Could you check a few things on this model? Use its own coordinates, in mm. Face numbers are marked on the shaded views. A direction names the side the tool comes from. Give positions to 0.01 mm unless a question says otherwise; leave off trailing zeros. Order: outer loops, then holes, each group sorted by start corner. A loop starts at its lowest first (then second) coordinate and runs counter-clockwise, first axis right, second up.
from build123d import *

# Parameters (mm, degrees)
SZKIC1_W                        = 27
SZKIC1_H                        = 25
ZAOKR_GLENIE1_R                 = 4
SZKIC4_R                        = 3
WYTNIJ_WYCI_GNI_CIE3_DEPTH      = 24.0000001
WYTNIJ_WYCI_GNI_CIE3_DEPTH_BACK = 3
WYTNIJ_WYCI_GNI_CIE2_DEPTH      = 24.0000001
SZKIC5_OUTSIDE_W                = 72.072
SZKIC5_OUTSIDE_H                = 72.072
WYTNIJ_WYCI_GNI_CIE4_DEPTH      = 26.0000001
SZKIC6_R                        = 2.675
WYTNIJ_WYCI_GNI_CIE5_DEPTH      = 26.0000001
SZKIC7_OUTSIDE_W                = 68.298
SZKIC7_OUTSIDE_H                = 29.798
WYTNIJ_WYCI_GNI_CIE6_DEPTH      = 5.5


with BuildPart() as part:
    # Szkic1 → Obrót1 (revolve)
    with BuildSketch(Plane.XY):
        with Locations((13.5, 12.5)):
            Rectangle(SZKIC1_W, SZKIC1_H)
    revolve(axis=Axis((0, 0, 0), (0, 1, 0)))

    # Szkic2 → Wycięcie-obrót1 (revolve, cut)
    with BuildSketch(Plane.XY):
        Polygon((5.55, 25), (5.55, 14.384163274), (27, 2), (27, 25), align=None)
    revolve(axis=Axis((0, 0, 0), (0, 1, 0)), mode=Mode.SUBTRACT)

    # Zaokrąglenie1
    zaokr_glenie1_edges = [part.edges().sort_by_distance(p)[0] for p in [
        (-5.55, 14.384163274, 0),
    ]]
    fillet(zaokr_glenie1_edges, radius=ZAOKR_GLENIE1_R)

    # Szkic4 → Wytnij-wyciągnięcie3 (cut, two sides)
    with BuildSketch(Plane(origin=(0, 2, 0), x_dir=(1, 0, 0), z_dir=(0, 1, 0))) as wytnij_wyci_gni_cie3_sk:
        with Locations((-20, 0)):
            Circle(SZKIC4_R)
        with Locations((20, 0)):
            Circle(SZKIC4_R)
    extrude(amount=WYTNIJ_WYCI_GNI_CIE3_DEPTH, mode=Mode.SUBTRACT)
    extrude(wytnij_wyci_gni_cie3_sk.sketch, amount=-WYTNIJ_WYCI_GNI_CIE3_DEPTH_BACK, mode=Mode.SUBTRACT)

    # Szkic3 → Wytnij-wyciągnięcie2 (cut, through all)
    with BuildSketch(Plane(origin=(0, 2, 0), x_dir=(1, 0, 0), z_dir=(0, 1, 0))):
        with BuildLine():
            Line((-17.5, 5), (-26.532998323, 5))
            ThreePointArc((-26.532998323, 5), (-27, 0), (-26.532998323, -5))
            Line((-26.532998323, -5), (-17.5, -5))
            ThreePointArc((-17.5, -5), (-12.5, 0), (-17.5, 5))
        make_face()
        with BuildLine():
            Line((17.5, 5), (26.532998323, 5))
            ThreePointArc((26.532998323, 5), (27, 0), (26.532998323, -5))
            Line((26.532998323, -5), (17.5, -5))
            ThreePointArc((17.5, -5), (12.5, 0), (17.5, 5))
        make_face()
    extrude(amount=WYTNIJ_WYCI_GNI_CIE2_DEPTH, mode=Mode.SUBTRACT)

    # Szkic5 outside → Wytnij-wyciągnięcie4 (cut, through all)
    with BuildSketch(Plane.XZ):
        Rectangle(SZKIC5_OUTSIDE_W, SZKIC5_OUTSIDE_H)
        with BuildLine():
            Line((-20.2625, 6.995076393), (-0.290625, 7.744548864))
            ThreePointArc((-0.290625, 7.744548864), (0, 7.75), (0.290625, 7.744548864))
            Line((0.290625, 7.744548864), (20.2625, 6.995076393))
            ThreePointArc((20.2625, 6.995076393), (27, 0), (20.2625, -6.995076393))
            Line((20.2625, -6.995076393), (0.290625, -7.744548864))
            ThreePointArc((0.290625, -7.744548864), (0, -7.75), (-0.290625, -7.744548864))
            Line((-0.290625, -7.744548864), (-20.2625, -6.995076393))
            ThreePointArc((-20.2625, -6.995076393), (-27, 0), (-20.2625, 6.995076393))
        make_face(mode=Mode.SUBTRACT)
    extrude(amount=-WYTNIJ_WYCI_GNI_CIE4_DEPTH, mode=Mode.SUBTRACT)

    # Szkic6 → Wytnij-wyciągnięcie5 (cut, through all)
    with BuildSketch(Plane(origin=(0, 25, 0), x_dir=(1, 0, 0), z_dir=(0, 1, 0))):
        Circle(SZKIC6_R)
    extrude(amount=-WYTNIJ_WYCI_GNI_CIE5_DEPTH, mode=Mode.SUBTRACT)

    # Szkic7 outside → Wytnij-wyciągnięcie6 (cut)
    with BuildSketch(Plane(origin=(0, 25, 0), x_dir=(1, 0, 0), z_dir=(0, 1, 0))):
        Rectangle(SZKIC7_OUTSIDE_W, SZKIC7_OUTSIDE_H)
        Polygon((-4.806440991, 2.775), (-4.806440991, -2.775), (0, -5.55), (4.806440991, -2.775), (4.806440991, 2.775), (0, 5.55), align=None, mode=Mode.SUBTRACT)
    extrude(amount=-WYTNIJ_WYCI_GNI_CIE6_DEPTH, mode=Mode.SUBTRACT)

    # Szkic9 → Wycięcie-obrót2 (revolve, cut)
    with BuildSketch(Plane.XY):
        Polygon((4.05, 25), (5.55, 24.133974596), (5.55, 25), align=None)
    revolve(axis=Axis((0, 19.5, 0), (0, 1, 0)), mode=Mode.SUBTRACT)


solid = part.part
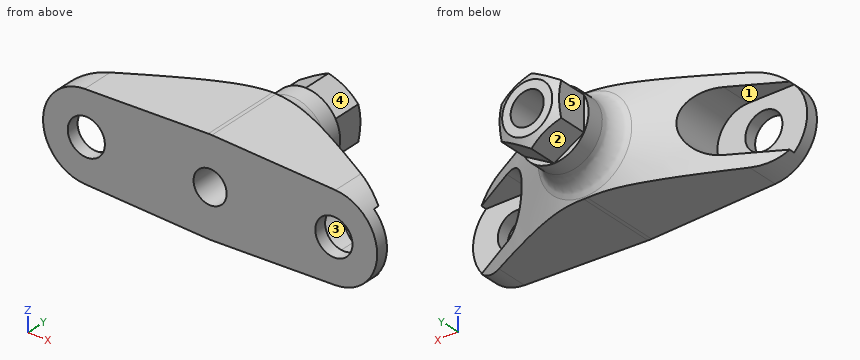
Item 1: For the marked faces 1, 2, 3, 4 and 5, which set-ups out of +Z, -Z, +X, -X, +Y, -Y let a thin tool reach every point of the face, with its end or its side?
Findings:
face 1: -X, +Y
face 2: -Z, -X, +Y
face 3: +X, +Y
face 4: +Z, +X, +Y
face 5: +Z, -Z, -X, +Y
Item 2: Imagine slicing it at B-B on z = 0. Give the number of separate pieces and of enclosed holes in the cut face, then the cut area to 3 significant figures.
Findings:
separate pieces: 4
enclosed holes: 0
area: 343 mm2
Item 3: Imagine slicing it at A-A on y = 21.25. List the corners of the cut face in (x, z) for me (3 decimals).
Findings:
outline: (-4.806, -2.775) - (0, -5.55) - (4.806, -2.775) - (4.806, 2.775) - (0, 5.55) - (-4.806, 2.775) - close; hole circle Ø5.35 at (0, 0)
Item 4: Please list where these lines run through material, in increasing order: line 1 along X through (y, z) = (1.15, 0) (3 decimals); line 2 along Z through (x, y) = (20, 0.7); line 3 along Y through (x, z) = (24, -0.75).
Findings:
line 1: x = -27 to -23, -17 to -2.675, 2.675 to 17, 23 to 27
line 2: z = -7 to -3, 3 to 7
line 3: y = 0 to 2
Item 5: For pin 1 (0.8 mm diameter, centred on x = 2.5, z = -4.5, fed in from +Y); pin 2 (1.4 mm diameter, centred on x = 3.5, z = 4, fed in from +Y); pin 3 (4 mm diameter, centred on x = -21.5, y = 5.5, fed in from -Z); pin 4 (1.5 mm diameter, centred on x = -19.5, z = -6, fed in from -Y), each with a flat end and sliding along its axis, tell me the tip position at first contact or that it passes through.
Findings:
pin 1: stops at y = 24.6
pin 2: stops at y = 24.67
pin 3: stops at z = -7.02
pin 4: stops at y = 0
